Here's how the part is built. I have some questions about the finished solid (model axes, mm). A direction names the side the tool comes from. Round coordinates to 2 decimals unless told otherwise and drop trailing zeros. Write each loop counter-clockwise with the first axis right and the second up, starting at its lowest first coordinate (ties: lowest second). Pieces come first, ordered by that corner, then holes. Notation, with made-up numbers: (71.25, -11.5) -> (77.25, -11.5) arc R17 ccw to (77.25, -3.5) -> close; hole circle Ø3 at (-0.75, 20.25). An arc over 180 degrees is marked (long way). Answer in a Markdown table with one row per item. Add a question column.
Autodesk Inventor part; units mm, degrees
ref_plane "YZ Plane" through (0, 0, 0) normal (1, 0, 0) x (0, 1, 0)
ref_plane "XZ Plane" through (0, 0, 0) normal (0, 1, 0) x (-1, 0, 0)
ref_plane "XY Plane" through (0, 0, 0) normal (0, 0, 1) x (1, 0, 0)
sketch "草圖1" plane through (0, 0, 0) normal (0, 0, 1) x (1, 0, 0)
  line L0 (-200, 0) -> (0, 0) construction
  line L1 (-200, -5) -> (0, -5)
  line L2 (0, 5) -> (-200, 5)
  arc A0 (-200, 5) -> (-200, -5) centre (-200, 0) ccw
  arc A1 (0, -5) -> (0, 5) centre (0, 0) ccw
  circle A2 centre (0, 0) radius 3.55
  circle A3 centre (-80, 0) radius 3.55
  circle A4 centre (-200, 0) radius 3.55
  point P0 (-100, 0)
  dimension "d0" = 200
  dimension "d1" = 10
  dimension "d3" = 7.1
  dimension "d27" = 7.1
  dimension "d47" = 7.1
extrude "擠出1" add sketch "草圖1" along normal blind 6 contours A0 L2 A1 L1 | A4
sketch "草圖4" plane through (0, 0, 0) normal (0, 0, -1) x (-1, 0, 0)
  line L0 (200, 0) -> (212, 0) construction
  line L1 (200, 8) -> (212, 8)
  line L2 (212, -8) -> (200, -8)
  arc A0 (200, 8) -> (200, -8) centre (200, 0) ccw
  arc A1 (212, -8) -> (212, 8) centre (212, 0) ccw
  circle A2 centre (200, 0) radius 3.4
  circle A3 centre (200, 0) radius 4.25
  circle A4 centre (216, 0) radius 0.6
  circle A5 centre (216, 0) radius 2.9
  circle A6 centre (200, 0) radius 6.2
  line L3 (216.3855, -2.8743) -> (204.265, -4.5)
  line L4 (216.3855, 2.8743) -> (204.265, 4.5)
  arc A7 (200, -5) -> (200, 5) centre (200, 0) ccw
  point P0 (0, 0)
  point P1 (206, 0)
  dimension "d31" = 8
  dimension "d32" = 8.5
  dimension "d33" = 6.8
  dimension "d34" = 12
  dimension "d36" = 1.2
  dimension "d37" = 16
  dimension "d42" = 5.8
  dimension "d44" = 12.4
  dimension "d46" = 9
extrude "擠出5" add sketch "草圖4" against normal blind 6 contours L1 A1 L2 A0 | A2 | A3 | A4 | A5 | A5 L3 A6 L4 | A6
extrude "擠出6" cut sketch "草圖4" against normal blind 3.35 contours A2 | A3 | A4 | A5 | A5 L3 A6 L4 | A6
extrude "擠出7" cut sketch "草圖1" along normal through all contours A4
sketch "草圖5" plane through (0, 0, 3.35) normal (0, 0, -1) x (-1, 0, 0)
  point P0 (0, 0)
properties part number "200_forservo"
Item 1: If we section it at B-B on z = 4.7: Please give me the cut outline in (x, y) (3 decimals), then the cut area to 3 significant figures.
Item 2: I need wall thicknesses on line 1 along X through (y, z) = (0.5, 5.7); line 2 along Y through (x, z) = (-200, 1.65); line 3 along Y through (x, z) = (-80, 2.25). Which ranges of each line are inside material? Lowest first, please. Write a range as from..to.
Item 3: If we section it at A-A on x = -80: Please give me the cut outline in (y, z), then the cut area to 3 significant figures.
Item 4: If we section it at D-D on x = -104: Please give me the cut outline in (y, z).
Item 5: For P1, Ø2, axis at x = -83, z = 2, coming from the +Y side; P2, Ø1.5, axis at x = -105.5, z = 5, coming from the -Y side, each with a flat end and sliding along its axis, tell me the tip position at first contact or that it passes through.
Item 6: On a 3-axis mill with a long thin cutter (end or side, diameter ignored), from which of +Z, -Z, +X, -X, +Y, -Y can I reach the whole of each face in a straight line? I mean faces 5 (the flat face through (-206, 8, 3)), 6 (the flat face through (-98, -5, 3)), 7 (the flat face through (-96, 5, 3)), 8 (the cylindrical face through (-0.46, -3.52, 2.96)), 9 (the flat face through (-206, 0, 3.35)). Say none if no direction works.
Item 7: If we mould it in two halves opening along X, with no side actions, what happens to faces 1 (the cylindrical face through (5, 0, 3)), 2 (the cylindrical face through (-220, 0, 3)), 3 (the flat face through (-206, -8, 3)), 4 (the cylindrical face through (-193.803, 0.202, 1.652))? For each: pulls with the +X half, pulls with the -X half, needs draft (parallel to the pull), parting line crosses it, or undercut.
Item 8: If we section it at C-C on y = 0: Please give me the cut outline in (x, z), then the cut area to 3 significant figures.
Results list:
| question | item | result |
|---|---|---|
| 1 | outline | (-212, -8) -> (-200, -8) arc R8 ccw to (-193.755, -5) -> (0, -5) arc R5 ccw to (0, 5) -> (-193.755, 5) arc R8 ccw to (-200, 8) -> (-212, 8) arc R8 ccw to start; hole circle Ø7.1 at (-200, 0); hole circle Ø7.1 at (-80, 0); hole circle Ø7.1 at (0, 0) |
| 1 | area | 2,240 mm² |
| 2 | line 1 | -219.98..-203.51, -196.49..-83.51, -76.49..-3.51, 3.51..4.97 |
| 2 | line 2 | -8..-6.2, 6.2..8 |
| 2 | line 3 | -5..-3.55, 3.55..5 |
| 3 | outline | (-5, 0) -> (-3.55, 0) -> (-3.55, 6) -> (-5, 6) -> close; (3.55, 0) -> (5, 0) -> (5, 6) -> (3.55, 6) -> close |
| 3 | area | 17.4 mm² |
| 4 | outline | (-5, 0) -> (5, 0) -> (5, 6) -> (-5, 6) -> close |
| 5 | P1 | y = 5 |
| 5 | P2 | y = -5 |
| 6 | face 5 | +Z, -Z, +X, -X, +Y |
| 6 | face 6 | +Z, -Z, +X, -Y |
| 6 | face 7 | +Z, -Z, +X, +Y |
| 6 | face 8 | +Z, -Z |
| 6 | face 9 | -Z |
| 7 | face 1 | pulls with the +X half |
| 7 | face 2 | pulls with the -X half |
| 7 | face 3 | needs draft |
| 7 | face 4 | undercut |
| 8 | outline | (-220, 0) -> (-218.9, 0) -> (-218.9, 3.35) -> (-203.55, 3.35) -> (-203.55, 6) -> (-220, 6) -> close; (-196.45, 3.35) -> (-193.8, 3.35) -> (-193.8, 0) -> (-83.55, 0) -> (-83.55, 6) -> (-196.45, 6) -> close; (-76.45, 0) -> (-3.55, 0) -> (-3.55, 6) -> (-76.45, 6) -> close; (3.55, 0) -> (5, 0) -> (5, 6) -> (3.55, 6) -> close |
| 8 | area | 1,160 mm² |
